Build history of the part. All positions in model axes, mm. A direction names the side the tool comes from. Give positions to 0.01 mm unless a question says otherwise; leave off trailing zeros. Loops run counter-clockwise (first coordinate to the right, second up) from the corner with the lowest first, then second, coordinate; pieces in that order, holes last. Notation, with made-up numbers: (-5, 13.25) - (26, 13.25) arc R19 ccw to (26, 33.25) - close; hole circle Ø5 at (-17, -24). An arc over 180 degrees is marked (long way). Return JSON: item names as keys, results as strings. Group by question number.
1) Slice it at B-B (x = 54.5). List the corners of the cut face in (y, z), and give its area (3 significant figures).
2) Slice it at D-D (x = -10). List the corners of the cut face in (y, z), and give its area (3 significant figures).
3) Slice it at C-C (z = 30). List the corners of the cut face in (x, y).
4) 3-axis set-ups, long thin cutter, end or side, ignore diameter. For faces 1 (the face through (15, -25, 2)), 2 (the face through (-15, -18, 29)), 3 (the face through (30, -5, 20)): which of +Z, -Z, +X, -X, +Y, -Y reach the whole face in a straight line?
5) Drill centre lines: probe 1 along Z at (x, y) = (-10, -84.25); probe 2 along Y at (x, z) = (-7.5, 39); probe 3 along Z at (x, y) = (-8.5, -85). Where is each one in solid material? Low to high. Write a range as from..to.
6) Mould opens along Z. For faces 4 (the face through (-10, -5, 80)), 5 (the face through (-20, -34, 23)), 6 (the face through (-11.075, -4.93, 66.686)) say: released by +Z, released by -Z, zero draft, split by the parting line, or undercut.
7) Drop flat-ended pins along their axis: pin 1 (24 mm diameter, centred on y = -22, z = 31, fed in from +X); pin 2 (12 mm diameter, centred on y = -32.5, z = 9.5, fed in from +X); pin 3 (6 mm diameter, centred on x = -6, y = -46, fed in from +Z); pin 4 (3.5 mm diameter, centred on x = -10, z = 30, fed in from -Y). Give the stop position or say it passes through.
8) Slice it at A-A (z = 10). List the corners of the cut face in (x, y).
```python
from build123d import *

# Parameters (mm, degrees)
F0_W      = 20
F0_H      = 20
F1_DEPTH  = 90
F2_W      = 20
F2_H      = 20
F2_W_2    = 60
F2_H_2    = 60
F3_DEPTH  = 10
F4_W      = 20
F4_H      = 60
F4_W_2    = 60
F4_H_2    = 20
F5_DEPTH  = 10
F6_R      = 2
F7_DEPTH  = 116.7
F9_DEPTH  = 5
F11_DEPTH = 5
F13_DEPTH = 5


with BuildPart() as f1:
    # F0 (on Front) → F1 (new body)
    with BuildSketch(Plane.XZ):
        with Locations((-10, 10)):
            Rectangle(F0_W, F0_H)
    extrude(amount=F1_DEPTH)

    # F2 (on face) → F3 (join)
    with BuildSketch(Plane.XZ.offset(90)):
        with Locations((-10, 10)):
            Rectangle(F2_W, F2_H)
        with Locations((30, 10)):
            Rectangle(F2_W_2, F2_H)
        with Locations((-10, 50)):
            Rectangle(F2_W, F2_H_2)
    extrude(amount=-F3_DEPTH)

    # F4 (on face) → F5 (join)
    with BuildSketch(Plane(origin=(0, 0, 0), x_dir=(-1, 0, 0), z_dir=(0, 1, 0))):
        with Locations((10, 50)):
            Rectangle(F4_W, F4_H)
        with Locations((-30, 10)):
            Rectangle(F4_W_2, F4_H_2)
    extrude(amount=-F5_DEPTH)

    # F6 (on face) → F7 (cut)
    with BuildSketch(Plane(origin=(0, 0, 0), x_dir=(-1, 0, 0), z_dir=(0, 1, 0))):
        with Locations((10, 65)):
            Circle(F6_R)
        with Locations((10, 30)):
            Circle(F6_R)
        with Locations((-45, 10)):
            Circle(F6_R)
        with Locations((-10, 10)):
            Circle(F6_R)
    extrude(amount=-F7_DEPTH, mode=Mode.SUBTRACT)

    # F8 (on face) → F9 (join)
    with BuildSketch(Plane.XZ.offset(90)):
        Polygon((0, 50), (0, 20), (30, 20), align=None)
    extrude(amount=-F9_DEPTH)

    # F10 (on face) → F11 (join)
    with BuildSketch(Plane(origin=(0, 0, 0), x_dir=(1, 0, 0), z_dir=(0, 0, -1))):
        Polygon((30, 80), (0, 80), (0, 50), align=None)
        Polygon((0, 10), (30, 10), (0, 40), align=None)
    extrude(amount=-F11_DEPTH)

    # F12 (on face) → F13 (join)
    with BuildSketch(Plane(origin=(-20, 0, 0), x_dir=(0, -1, 0), z_dir=(-1, 0, 0))):
        Polygon((10, 50), (10, 20), (40, 20), align=None)
        Polygon((80, 20), (80, 50), (50, 20), align=None)
    extrude(amount=-F13_DEPTH)


solid = f1.part
```
Results:
{
 "1": {"outline": "(-90, 0) - (-80, 0) - (-80, 20) - (-90, 20) - close; (-10, 0) - (0, 0) - (0, 20) - (-10, 20) - close", "area": "400 mm2"},
 "2": {"outline": "(-90, 0) - (0, 0) - (0, 28) - (-10, 28) - (-10, 20) - (-80, 20) - (-80, 28) - (-90, 28) - close; (-90, 32) - (-80, 32) - (-80, 63) - (-90, 63) - close; (-90, 67) - (-80, 67) - (-80, 80) - (-90, 80) - close; (-10, 32) - (0, 32) - (0, 63) - (-10, 63) - close; (-10, 67) - (0, 67) - (0, 80) - (-10, 80) - close", "area": "2,840 mm2"},
 "3": {"outline": "(-20, -90) - (-12, -90) - (-12, -80) - (-15, -80) - (-15, -60) - (-20, -60) - close; (-20, -30) - (-15, -30) - (-15, -10) - (-12, -10) - (-12, 0) - (-20, 0) - close; (-8, -90) - (20, -90) - (20, -85) - (0, -85) - (0, -80) - (-8, -80) - close; (-8, -10) - (0, -10) - (0, 0) - (-8, 0) - close"},
 "4": {"face 1": "+Z, -Z, +X", "face 2": "+Z, +X", "face 3": "+Z, +X, +Y"},
 "5": {"probe 1": "0..28, 32..63, 67..80", "probe 2": "-90..-80, -10..0", "probe 3": "0..28.68, 31.32..63.68, 66.32..80"},
 "6": {"face 4": "released by +Z", "face 5": "zero draft", "face 6": "undercut"},
 "7": {"pin 1": "x = 0", "pin 2": "x = 11.47", "pin 3": "z = 20", "pin 4": "through"},
 "8": {"outline": "(-20, -90) - (8, -90) - (8, -80) - (0, -80) - (0, -10) - (8, -10) - (8, 0) - (-20, 0) - close; (12, -90) - (43, -90) - (43, -80) - (12, -80) - close; (12, -10) - (43, -10) - (43, 0) - (12, 0) - close; (47, -90) - (60, -90) - (60, -80) - (47, -80) - close; (47, -10) - (60, -10) - (60, 0) - (47, 0) - close"}
}
